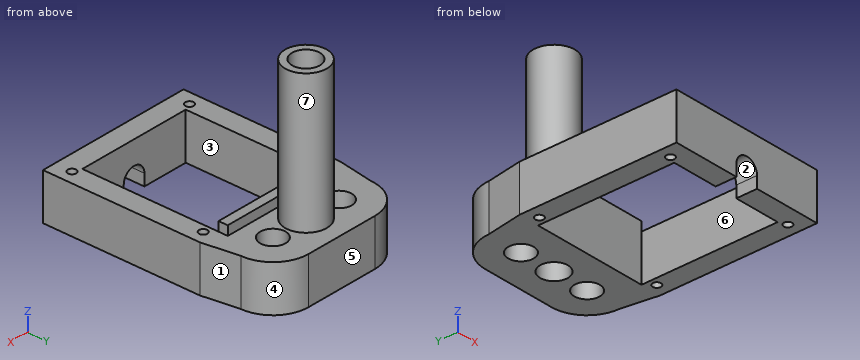
```python
from build123d import *

# Parameters (mm, degrees)
SKETCH1_R           = 2.75
BOSS_EXTRUDE1_DEPTH = 10
SKETCH2_R           = 3
CUT_EXTRUDE1_DEPTH  = 15
SKETCH3_R           = 4.5
SKETCH3_R_2         = 3
BOSS_EXTRUDE2_DEPTH = 30
BOSS_EXTRUDE4_DEPTH = 10
CUT_EXTRUDE2_DEPTH  = 10
SKETCH7_W           = 25
SKETCH7_H           = 2
BOSS_EXTRUDE6_DEPTH = 2
SKETCH8_R           = 0.9
CUT_EXTRUDE3_DEPTH  = 19


with BuildPart() as part:
    # Sketch1 → Boss-Extrude1 (new body)
    with BuildSketch(Plane.XY):
        with BuildLine():
            Line((8, 7.75), (-8, 7.75))
            ThreePointArc((-8, 7.75), (-15.75, 0), (-8, -7.75))
            Line((-8, -7.75), (8, -7.75))
            ThreePointArc((8, -7.75), (15.75, 0), (8, 7.75))
        make_face()
        with Locations((-8, 0)):
            Circle(SKETCH1_R, mode=Mode.SUBTRACT)
        with Locations((8, 0)):
            Circle(SKETCH1_R, mode=Mode.SUBTRACT)
    extrude(amount=BOSS_EXTRUDE1_DEPTH)

    # Sketch2 → Cut-Extrude1 (cut)
    with BuildSketch(Plane.XY.offset(10)):
        Circle(SKETCH2_R)
    extrude(amount=-CUT_EXTRUDE1_DEPTH, mode=Mode.SUBTRACT)

    # Sketch3 → Boss-Extrude2 (add)
    with BuildSketch(Plane.XY.offset(10)):
        Circle(SKETCH3_R)
        Circle(SKETCH3_R_2, mode=Mode.SUBTRACT)
    extrude(amount=BOSS_EXTRUDE2_DEPTH)

    # Sketch5 → Boss-Extrude4 (add)
    with BuildSketch(Plane.XY):
        Polygon((-12.5, -7.75), (-17, -7.75), (-17, -41.75), (17, -41.75), (17, -7.75), (12.5, -7.75), (12.5, -12.25), (12.5, -37.25), (-12.5, -37.25), (-12.5, -12.25), align=None)
        with BuildLine():
            ThreePointArc((-8, -7.75), (-13.480077554, -5.480077554), (-15.75, 0))
            Line((-15.75, 0), (-17, -7.75))
            Line((-17, -7.75), (-12.5, -7.75))
            Line((-12.5, -7.75), (-8, -7.75))
        make_face()
        with BuildLine():
            ThreePointArc((15.75, 0), (13.480077554, -5.480077554), (8, -7.75))
            Line((8, -7.75), (12.5, -7.75))
            Line((12.5, -7.75), (17, -7.75))
            Line((17, -7.75), (15.75, 0))
        make_face()
    extrude(amount=BOSS_EXTRUDE4_DEPTH)

    # Sketch6 → Cut-Extrude2 (cut)
    with BuildSketch(Plane.XZ.offset(41.75)):
        with BuildLine():
            Line((-2.5, 0), (2.5, 0))
            Line((2.5, 0), (2.5, 2.5))
            ThreePointArc((2.5, 2.5), (0, 5), (-2.5, 2.5))
            Line((-2.5, 2.5), (-2.5, 0))
        make_face()
    extrude(amount=-CUT_EXTRUDE2_DEPTH, mode=Mode.SUBTRACT)

    # Sketch7 → Boss-Extrude6 (add)
    with BuildSketch(Plane.XY.offset(10)):
        with Locations((0, -6.75)):
            Rectangle(SKETCH7_W, SKETCH7_H)
    extrude(amount=BOSS_EXTRUDE6_DEPTH)

    # Sketch8 → Cut-Extrude3 (cut)
    with BuildSketch(Plane.XY.offset(10)):
        with Locations((-14.2, -9.55)):
            Circle(SKETCH8_R)
        with Locations((14.2, -9.55)):
            Circle(SKETCH8_R)
        with Locations((14.2, -37.95)):
            Circle(SKETCH8_R)
        with Locations((-14.2, -37.95)):
            Circle(SKETCH8_R)
    extrude(amount=-CUT_EXTRUDE3_DEPTH, mode=Mode.SUBTRACT)


solid = part.part
```
Here's how the part is built. I have some questions about the finished solid (model axes, mm). Face numbers are marked on the shaded views. A direction names the side the tool comes from. Coordinates: 2 decimals unless noted, no trailing zeros. Order: outer loops, then holes, each group sorted by start corner. A loop starts at its lowest first (then second) coordinate and runs counter-clockwise, first axis right, second up.
Item 1: If we section it at A-A, the plane y = -37.95: List the corners of the cut face in (x, z) for me.
Response values:
outline: (-17, 0) - (-15.1, 0) - (-15.1, 10) - (-17, 10) - close; (-13.3, 0) - (-2.5, 0) - (-2.5, 2.5) arc R2.5 cw to (2.5, 2.5) - (2.5, 0) - (13.3, 0) - (13.3, 10) - (-13.3, 10) - close; (15.1, 0) - (17, 0) - (17, 10) - (15.1, 10) - close
Item 2: If we section it at B-B, the plane x = 14.2: List the corners of the cut face in (y, z) for me, then the cut area to 3 significant figures.
Response values:
outline: (-41.75, 0) - (-38.85, 0) - (-38.85, 10) - (-41.75, 10) - close; (-37.05, 0) - (-10.45, 0) - (-10.45, 10) - (-37.05, 10) - close; (-8.65, 0) - (4.65, 0) - (4.65, 10) - (-8.65, 10) - close
area: 428 mm2
Item 3: I'm going to push flat-ended pins straight in: pin 1 Ø0.6 at (x, y) = (-1.5, -6.5) entering from +Z; pin 2 Ø1 at (x, z) = (2, 33.5) entering from -Y; pin 3 Ø1.6 at (y, z) = (-7, 11.5) entering from +X; pin 4 Ø3.5 at (x, y) = (-8, 0) entering from -Z. Where does each tip first touch, or does it pass through?
Response values:
pin 1: stops at z = 12
pin 2: stops at y = -4.24
pin 3: stops at x = 12.5
pin 4: passes through
Item 4: Which directions (+Z, -Z, +X, -X, +Y, -Y) give clear straight access to the entire face, cutting with the end or side of a thin tool? Please do the marked faces 1, 2 and 3.
Response values:
face 1: +Z, -Z, +X, +Y
face 2: -Z, -Y
face 3: +Z, -Z
Item 5: Thinking about a two-plate mould opening in X: for the marked faces 4, 5, 6 and 7, which applies, pulls with the +X half, pulls with the -X half, needs draft (parallel to the pull), parting line crosses it, or undercut?
Response values:
face 4: pulls with the +X half
face 5: needs draft
face 6: undercut
face 7: parting line crosses it
Item 6: I need wall thicknesses on probe 1 along Y at (x, z) = (0, 26.75); probe 2 along X at (y, z) = (-14.5, 6); probe 3 along X at (y, z) = (-9, 8). Which ranges of each line are inside material? Lowest first, please.
Response values:
probe 1: y = -4.5 to -3, 3 to 4.5
probe 2: x = -17 to -12.5, 12.5 to 17
probe 3: x = -17 to -14.91, -13.49 to -12.5, 12.5 to 13.49, 14.91 to 17
Item 7: If we section it at C-C, the plane y = -26: List the corners of the cut face in (x, z) for me, then the cut area to 3 significant figures.
Response values:
outline: (-17, 0) - (-12.5, 0) - (-12.5, 10) - (-17, 10) - close; (12.5, 0) - (17, 0) - (17, 10) - (12.5, 10) - close
area: 90.0 mm2
Item 8: If we section it at D-D, the plane y = -9.55: List the corners of the cut face in (x, z) for me, then the cut area to 3 significant figures.
Response values:
outline: (-17, 0) - (-15.1, 0) - (-15.1, 10) - (-17, 10) - close; (-13.3, 0) - (-12.5, 0) - (-12.5, 10) - (-13.3, 10) - close; (12.5, 0) - (13.3, 0) - (13.3, 10) - (12.5, 10) - close; (15.1, 0) - (17, 0) - (17, 10) - (15.1, 10) - close
area: 54.0 mm2
